from build123d import *

# Parameters (mm, degrees)
MODEL_W             = 5.5
MODEL_H             = 5.5
BOSS_EXTRUDE1_DEPTH = 6


with BuildPart() as part:
    # Model → Boss-Extrude1 (new body)
    with BuildSketch(Plane.XY):
        with BuildLine():
            Line((3321.525540583, 1259.877349699), (3321.525540583, 1256.877349699))
            Line((3321.525540583, 1256.877349699), (3334.025540583, 1256.877349699))
            Line((3334.025540583, 1256.877349699), (3334.025540583, 1250.877349699))
            Line((3334.025540583, 1250.877349699), (3340.025540583, 1250.877349699))
            Line((3340.025540583, 1250.877349699), (3340.025540583, 1256.877349699))
            Line((3340.025540583, 1256.877349699), (3342.525540583, 1256.877349699))
            Line((3342.525540583, 1256.877349699), (3342.525540583, 1287.823726924))
            ThreePointArc((3342.525540583, 1287.823726924), (3372.525540583, 1300.877349699), (3402.525540583, 1287.823726924))
            Line((3402.525540583, 1287.823726924), (3402.525540583, 1256.877349699))
            Line((3402.525540583, 1256.877349699), (3413.525540583, 1256.877349699))
            Line((3413.525540583, 1256.877349699), (3423.525540583, 1256.877349699))
            Line((3423.525540583, 1256.877349699), (3423.525540583, 1259.877349699))
            ThreePointArc((3423.525540583, 1259.877349699), (3372.525540583, 1310.877349699), (3321.525540583, 1259.877349699))
        make_face()
        with Locations((3408.025540583, 1262.377349699)):
            Rectangle(MODEL_W, MODEL_H, mode=Mode.SUBTRACT)
        with Locations((3408.025540583, 1282.377349699)):
            Rectangle(MODEL_W, MODEL_H, mode=Mode.SUBTRACT)
        with Locations((3337.025540583, 1262.377349699)):
            Rectangle(MODEL_W, MODEL_H, mode=Mode.SUBTRACT)
        with Locations((3337.025540583, 1282.377349699)):
            Rectangle(MODEL_W, MODEL_H, mode=Mode.SUBTRACT)
    extrude(amount=BOSS_EXTRUDE1_DEPTH)


solid = part.part
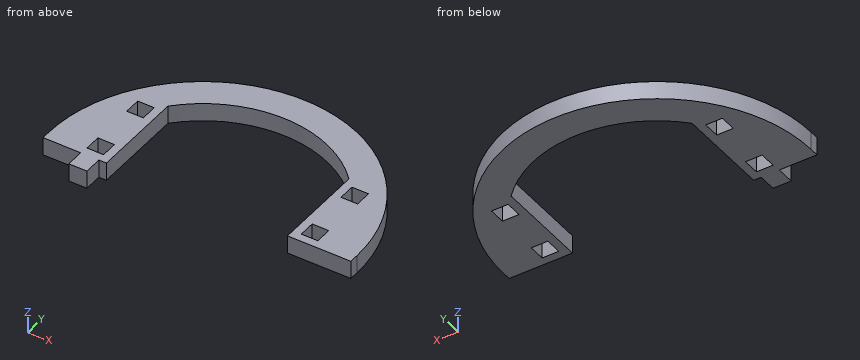
Geometry: final body of the model. Coordinates: model frame, mm. Coordinates: 2 decimals unless noted, no trailing zeros. Order: outer loops, then holes, each group sorted by start corner. A loop starts at its lowest first (then second) coordinate and runs counter-clockwise, first axis right, second up.
(1) First-contact query: pin 1 (3 mm diameter, centred on y = 1253.5, z = 4.5, fed in from -X); pin 2 (1.8 mm diameter, centred on y = 1277.5, z = 2.5, fed in from -X); pin 3 (3 mm diameter, centred on x = 3411.5, z = 2, fed in from -Y); pin 4 (4 mm diameter, centred on x = 3412.5, y = 1297, fed in from +Z). Flat tips, straight axial feed; report the tip coordinate or a pass-through.
(2) Section query B-B (z = 2.1). Return the cut outline in (x, y), plus the area to 3 significant figures.
(3) Section query C-C (x = 3337.5). Return the cut outline in (y, z).
(4) Section query A-A (y = 1258). Return the cut outline in (x, z).
(5) Material intervals for probe 1 along X at (y, z) = (1260, 0.6); probe 2 along Y at (x, z) = (3409, 4.65); probe 3 along X at (y, z) = (1257.5, 5.35), sorted ascending.
(6) Section query D-D (y = 1297). Return the cut outline in (x, z), plus the area to 3 significant figures.
Solution:
1. pin 1: stops at x = 3334.03
1. pin 2: stops at x = 3324.35
1. pin 3: stops at y = 1256.88
1. pin 4: passes through
2. outline: (3321.53, 1256.88) - (3334.03, 1256.88) - (3334.03, 1250.88) - (3340.03, 1250.88) - (3340.03, 1256.88) - (3342.53, 1256.88) - (3342.53, 1287.82) arc R41 cw to (3402.53, 1287.82) - (3402.53, 1256.88) - (3423.53, 1256.88) - (3423.53, 1259.88) arc R51 ccw to (3321.53, 1259.88) - close; hole (3334.28, 1259.63) - (3339.78, 1259.63) - (3339.78, 1265.13) - (3334.28, 1265.13) - close; hole (3334.28, 1279.63) - (3339.78, 1279.63) - (3339.78, 1285.13) - (3334.28, 1285.13) - close; hole (3405.28, 1259.63) - (3410.78, 1259.63) - (3410.78, 1265.13) - (3405.28, 1265.13) - close; hole (3405.28, 1279.63) - (3410.78, 1279.63) - (3410.78, 1285.13) - (3405.28, 1285.13) - close
2. area: 1,910 mm2
3. outline: (1250.88, 0) - (1259.63, 0) - (1259.63, 6) - (1250.88, 6) - close; (1265.13, 0) - (1279.63, 0) - (1279.63, 6) - (1265.13, 6) - close; (1285.13, 0) - (1296.95, 0) - (1296.95, 6) - (1285.13, 6) - close
4. outline: (3321.53, 0) - (3342.53, 0) - (3342.53, 6) - (3321.53, 6) - close; (3402.53, 0) - (3423.53, 0) - (3423.53, 6) - (3402.53, 6) - close
5. probe 1: x = 3321.53 to 3334.28, 3339.78 to 3342.53, 3402.53 to 3405.28, 3410.78 to 3423.53
5. probe 2: y = 1256.88 to 1259.63, 1265.13 to 1279.63, 1285.13 to 1295.52
5. probe 3: x = 3321.53 to 3342.53, 3402.53 to 3423.53
6. outline: (3337.56, 0) - (3355.12, 0) - (3355.12, 6) - (3337.56, 6) - close; (3389.93, 0) - (3407.5, 0) - (3407.5, 6) - (3389.93, 6) - close
6. area: 211 mm2
